Autodesk Inventor part; units mm, degrees
ref_plane "YZ Plane" through (0, 0, 0) normal (1, 0, 0) x (0, 1, 0)
ref_plane "XZ Plane" through (0, 0, 0) normal (0, 1, 0) x (-1, 0, 0)
ref_plane "XY Plane" through (0, 0, 0) normal (0, 0, 1) x (1, 0, 0)
sketch "Sketch1" plane through (0, 0, 0) normal (0, 0, 1) x (1, 0, 0)
  circle A0 centre (0, 0) radius 10
  line L0 (0, 10) -> (0, 8)
  line L1 (0, -10) -> (0, -8)
  line L2 (-6, -8) -> (6, -8)
  line L3 (-6, 8) -> (6, 8)
  point P0 (-6, 8)
  point P1 (-6, -8)
  dimension "d0" = 20
  dimension "d28" = 2
  dimension "d29" = 2
extrude "Extrusion1" add sketch "Sketch1" against normal blind 12 contours A0 L2 L3
hole "Hole1" at (0, 0, 0) direction (0, 0, -1) diameter 10 depth 6
hole "Hole2" at (0, 0, 0) direction (0, 0, -1) diameter 6 end through all
thread "Thread1"
thread "Thread2"
chamfer "Chamfer3" distance 0.5 angle 45 8 edges at (0, 8, 0) (0, -8, 0) (10, 0, 0) (-10, 0, 0) (0, -8, -12) (0, 8, -12) (10, 0, -12) (-10, 0, -12)
chamfer "Chamfer4" distance 0.5 angle 45 2 edges at (0, 5, 0) (0, 3, -12)
properties part number "NozzleConnector"
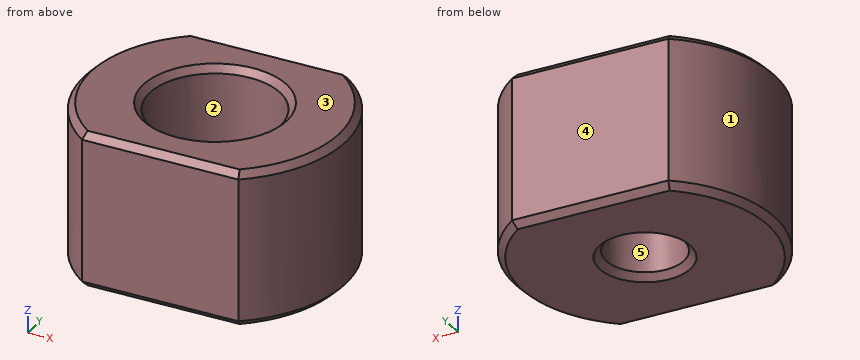
Geometry check sheet. Reference: the model listing, model coordinates, mm. Face numbers are marked on the shaded views. A direction names the side the tool comes from. Give positions to 0.01 mm unless a question says otherwise; leave off trailing zeros. Order: outer loops, then holes, each group sorted by start corner. A loop starts at its lowest first (then second) coordinate and runs counter-clockwise, first axis right, second up.
1. Sectioned sample at B-B (y = 0). Record the boundary of the cut face in (x, z), then the cut area to 3 significant figures.
Completed:
outline: (-10, -11.5) - (-9.5, -12) - (-3.5, -12) - (-3, -11.5) - (-3, -6) - (-5, -6) - (-5, -0.5) - (-5.5, 0) - (-9.5, 0) - (-10, -0.5) - close; (3, -11.5) - (3.5, -12) - (9.5, -12) - (10, -11.5) - (10, -0.5) - (9.5, 0) - (5.5, 0) - (5, -0.5) - (5, -6) - (3, -6) - close
area: 143 mm2
2. Sectioned sample at D-D (z = -1.25). Record the boundary of the cut face in (x, y).
Completed:
outline: (-6, -8) - (6, -8) arc R10 ccw to (6, 8) - (-6, 8) arc R10 ccw to start; hole circle Ø10 at (0, 0)
3. Depth check by flat-ended pin: pin 1 (3 mm diameter, centred on y = 6, z = -5, fed in from -X); pin 2 (2 mm diameter, centred on y = 2, z = -6, fed in from +X); pin 3 (3 mm diameter, centred on y = 5.5, z = -3.5, fed in from -X). Enter the tip coordinate at first touch or a pass-through.
Completed:
pin 1: stops at x = -8.93
pin 2: stops at x = 9.95
pin 3: stops at x = -9.17
4. Access from +Z, -Z, +X, -X, +Y, -Y to the whole of each face (thin tool, end or side, straight path). Record for the marked faces 1 and 2.
Completed:
face 1: +Z, -Z, -X
face 2: +Z
5. Scan lines: line 1 (Y direction, x = 0, z = -8.15); line 2 (Y direction, x = 0, z = -2.2); line 3 (X direction, y = -4, z = -5). Record each from-to range of solid material in increasing order.
Completed:
line 1: y = -8 to -3, 3 to 8
line 2: y = -8 to -5, 5 to 8
line 3: x = -9.17 to -3, 3 to 9.17
6. Sectioned sample at C-C (z = -7.5). Record the boundary of the cut face in (x, y), then the cut area to 3 significant figures.
Completed:
outline: (-6, -8) - (6, -8) arc R10 ccw to (6, 8) - (-6, 8) arc R10 ccw to start; hole circle Ø6 at (0, 0)
area: 253 mm2
7. Draft check along Y on the marked faces 3, 4 and 5. Enter one of: pulls with the +Y half, pulls with the -Y half, needs draft (parallel to the pull), parting line crosses it, or undercut.
Completed:
face 3: needs draft
face 4: pulls with the +Y half
face 5: undercut
8. Sectioned sample at A-A (x = 0). Record the boundary of the cut face in (y, z), then the cut area to 3 significant figures.
Completed:
outline: (-8, -11.5) - (-7.5, -12) - (-3.5, -12) - (-3, -11.5) - (-3, -6) - (-5, -6) - (-5, -0.5) - (-5.5, 0) - (-7.5, 0) - (-8, -0.5) - close; (3, -11.5) - (3.5, -12) - (7.5, -12) - (8, -11.5) - (8, -0.5) - (7.5, 0) - (5.5, 0) - (5, -0.5) - (5, -6) - (3, -6) - close
area: 95.0 mm2
